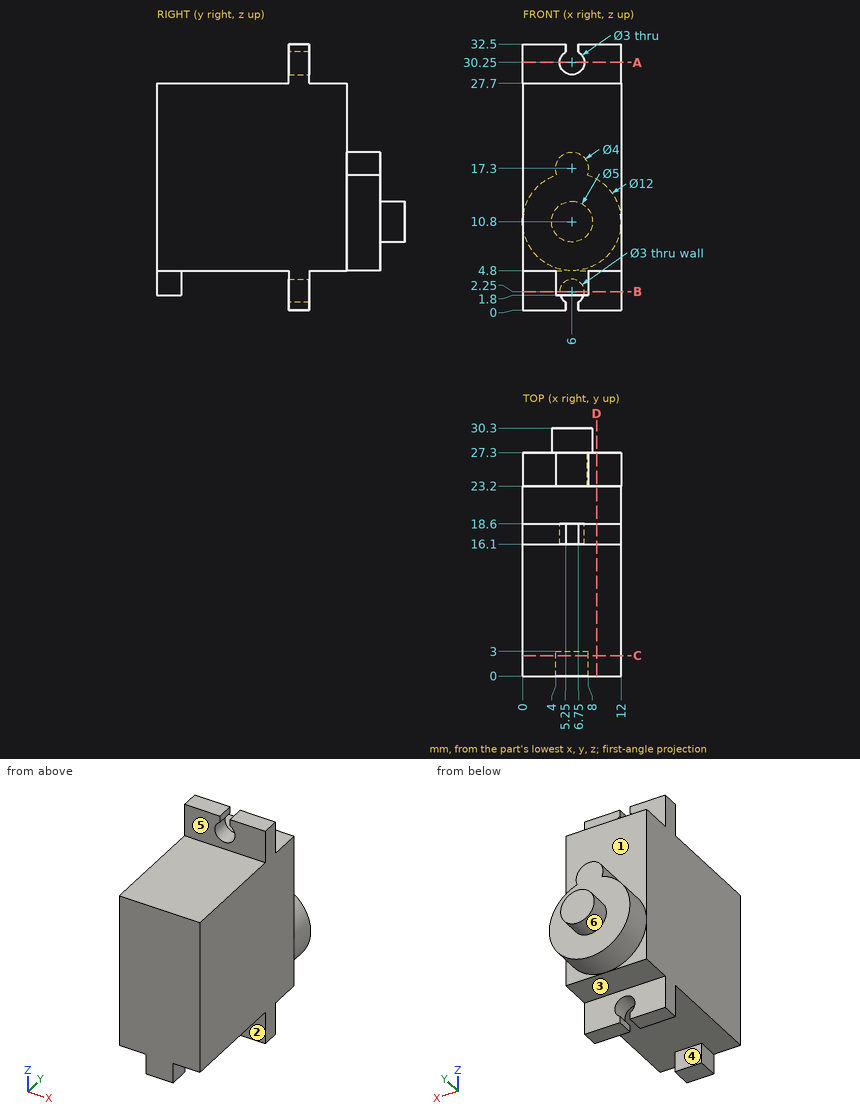
For this review, use the dimensioned drawing (mm, ordinates from the lowest corner) and the shaded views. A direction names the side the tool comes from. Coordinates: 2 decimals unless noted, no trailing zeros. Order: outer loops, then holes, each group sorted by start corner. A loop starts at its lowest first (then second) coordinate and runs counter-clockwise, first axis right, second up. Notation, with made-up numbers: (-2.75, 28) - (39.25, 28) arc R29 ccw to (39.25, 63) - close; hole circle Ø5 at (-27.5, 39.25). An arc over 180 degrees is marked (long way). Answer as a JSON object with one key per item and string values. Group by question number.
1. We need section C-C on y = 2.5. State the section outline as (x, z) points.
2. We need section A-A on z = 30.25. State the section outline as (x, y) points, then the cut area to 3 significant figures.
3. The part is to be moulded in two halves that separate along Y. For the marked faces 1, 2 and 3, say which applies: pulls with the +Y half, pulls with the -Y half, needs draft (parallel to the pull), parting line crosses it, or undercut.
4. For the marked faces 4, 5 and 6, list the 3-axis set-ups (+Z, -Z, +X, -X, +Y, -Y) from which the entire face can be reached by the end or side of a thin tool; tool diameter is ignored.
5. We need section D-D on x = 9. State the section outline as (y, z) points, then the cut area to 3 significant figures.
6. For probe 1 along Y at (x, z) = (5.5, 4); probe 2 along X at (y, z) = (16.85, 2.25); probe 3 along Y at (x, z) = (4, 23), list the stretches that pass through material, from the lowest coordinate up.
7. Clearance check with flat-ended pins moving along their axes: P1, Ø4, axis at x = 4, z = 3.5, coming from the -Y side; P2, Ø1.4, axis at x = 3.5, z = 29, coming from the -Y side; P3, Ø3, axis at x = 8.5, y = 4, coming from the +Z side; P4, Ø4, axis at x = 3.5, z = 23, coming from the +Y side. State where each tip first meets the part, or that it passes through.
8. We need section B-B on z = 2.25. State the section outline as (x, y) points.
Final values:
{
 "1": {"outline": "(0, 4.8) - (4, 4.8) - (4, 1.8) - (8, 1.8) - (8, 4.8) - (12, 4.8) - (12, 27.7) - (0, 27.7) - close"},
 "2": {"outline": "(0, 16.1) - (4.5, 16.1) - (4.5, 18.6) - (0, 18.6) - close; (7.5, 16.1) - (12, 16.1) - (12, 18.6) - (7.5, 18.6) - close", "area": "22.5 mm²"},
 "3": {"face 1": "pulls with the +Y half", "face 2": "undercut", "face 3": "needs draft"},
 "4": {"face 4": "-Z, +X, -X", "face 5": "+Z, +X, -X, -Y", "face 6": "+Y"},
 "5": {"outline": "(0, 4.8) - (16.1, 4.8) - (16.1, 0) - (18.6, 0) - (18.6, 4.8) - (23.2, 4.8) - (23.2, 5.6) - (27.3, 5.6) - (27.3, 16) - (23.2, 16) - (23.2, 27.7) - (18.6, 27.7) - (18.6, 32.5) - (16.1, 32.5) - (16.1, 27.7) - (0, 27.7) - close", "area": "598 mm²"},
 "6": {"probe 1": "0 to 3, 16.1 to 18.6", "probe 2": "0 to 4.5, 7.5 to 12", "probe 3": "0 to 23.2"},
 "7": {"P1": "y = 0", "P2": "y = 16.1", "P3": "z = 27.7", "P4": "y = 23.2"},
 "8": {"outline": "(0, 16.1) - (4.5, 16.1) - (4.5, 18.6) - (0, 18.6) - close; (4, 0) - (8, 0) - (8, 3) - (4, 3) - close; (7.5, 16.1) - (12, 16.1) - (12, 18.6) - (7.5, 18.6) - close"}
}
